Read the model definition and answer for the solid it produces. Units are mm, in the model's axes. Face numbers are marked on the shaded views. A direction names the side the tool comes from. Coordinates: 2 decimals unless noted, no trailing zeros. Loops run counter-clockwise (first coordinate to the right, second up) from the corner with the lowest first, then second, coordinate; pieces in that order, holes last. Notation, with made-up numbers: (-15.75, 6.5) - (41.25, 6.5) arc R8 cw to (41.25, 17.5) - close; hole circle Ø6 at (-11, 42). An arc over 180 degrees is marked (long way). Use one line per item in the form item = value. Start each with the question number.
1) A cutting plane is placed at A-A (z = 0). Give the vertices of the cut face in (x, y), and give its area (3 significant figures).
2) A cutting plane is placed at C-C (z = -12). Give the vertices of the cut face in (x, y).
3) Consider line 1 (X direction, y = -5.5, z = -16.5); line 2 (Z direction, x = 0, y = 1.4); line 3 (Y direction, x = 13, z = -13). Determine where each line is inside the solid, lowest interval first.
4) A cutting plane is placed at D-D (x = -5). Give the vertices of the cut face in (y, z), and give its area (3 significant figures).
5) A cutting plane is placed at B-B (y = -2). Give the vertices of the cut face in (x, z).
6) The mould has two halves that part along X. Classify the marked faces 1, 2, 3 and 4: released by +X, released by -X, zero draft, split by the parting line, or undercut.
7) Which of the six approach directions +Z, -Z, +X, -X, +Y, -Y give full straight-line access (tool end or side, diameter ignored) to the marked faces 5 and 6?
8) Each of these flat-tipped pins is pushed along its axis until it touches: P1, Ø2.5, axis at x = 14, z = -13, coming from the -Y side; P2, Ø4.5, axis at x = -13, y = -5.5, coming from the -Z side. Where does it stop, or does it pass through?
from build123d import *

# Parameters (mm, degrees)
F0_W     = 36
F0_H     = 37
F0_R     = 15
F1_DEPTH = 14
F0_R_2   = 12.5
F2_DEPTH = 3
F3_R     = 1.65
F4_DEPTH = 5
F5_R     = 2.5
F6_DEPTH = 8


with BuildPart() as f1:
    # F0 (on Front) → F1 (new body)
    with BuildSketch(Plane.XZ):
        with Locations((0, -0.5)):
            Rectangle(F0_W, F0_H)
        Circle(F0_R, mode=Mode.SUBTRACT)
    extrude(amount=F1_DEPTH)

    # F0 (on Front) → F2 (join)
    with BuildSketch(Plane.XZ):
        with Locations((0, -0.5)):
            Rectangle(F0_W, F0_H)
        Circle(F0_R, mode=Mode.SUBTRACT)
        Circle(F0_R)
        Circle(F0_R_2, mode=Mode.SUBTRACT)
    extrude(amount=-F2_DEPTH)

    # F3 (on face) → F4 (cut)
    with BuildSketch(Plane.XZ.offset(14)):
        with Locations((-14, 13)):
            Circle(F3_R)
        with Locations((-14, -13)):
            Circle(F3_R)
        with Locations((14, -13)):
            Circle(F3_R)
        with Locations((14, 13)):
            Circle(F3_R)
    extrude(amount=-F4_DEPTH, mode=Mode.SUBTRACT)

    # F5 (on face) → F6 (cut)
    with BuildSketch(Plane(origin=(0, 0, -19), x_dir=(1, 0, 0), z_dir=(0, 0, -1))):
        with Locations((-13, 5.5)):
            Circle(F5_R)
        with Locations((13, 5.5)):
            Circle(F5_R)
    extrude(amount=-F6_DEPTH, mode=Mode.SUBTRACT)


solid = f1.part
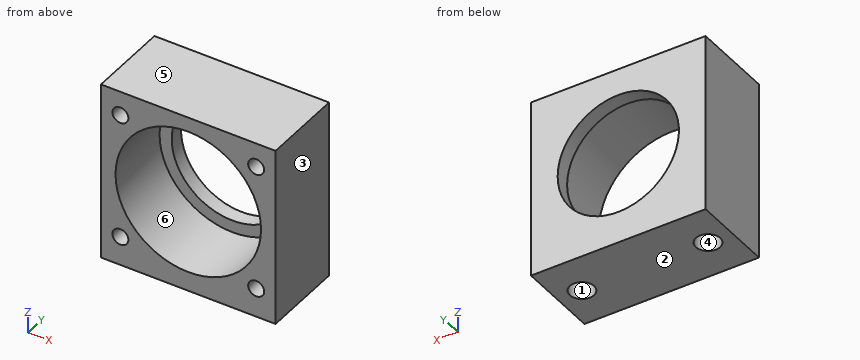
Found:
q1.outline = (-18, -14) - (-15, -14) - (-15, 0) - (-12.5, 0) - (-12.5, 3) - (-18, 3) - close; (12.5, 0) - (15, 0) - (15, -14) - (18, -14) - (18, 3) - (12.5, 3) - close
q1.area = 117 mm^2
q2.outline = (-18, -14) - (-15.31, -14) - (-15.31, -9) - (-12.69, -9) - (-12.69, -14) - (-9, -14) - (-9, 0) - (-3.5, 0) - (-3.5, 3) - (-18, 3) - close; (3.5, 0) - (9, 0) - (9, -14) - (12.69, -14) - (12.69, -9) - (15.31, -9) - (15.31, -14) - (18, -14) - (18, 3) - (3.5, 3) - close; hole circle Ø5 at (-13, -5.5); hole circle Ø5 at (13, -5.5)
q3.line_1 = -18 to -15.5, -10.5 to 10.5, 15.5 to 18
q3.line_2 = -19 to -12.5, 12.5 to 18
q3.line_3 = -9 to -8, -3 to 3
q4.outline = (-14, -19) - (3, -19) - (3, -11.46) - (0, -11.46) - (0, -14.14) - (-14, -14.14) - close; (-14, 14.14) - (0, 14.14) - (0, 11.46) - (3, 11.46) - (3, 18) - (-14, 18) - close
q4.area = 164 mm^2
q5.outline = (-18, -19) - (18, -19) - (18, 18) - (-18, 18) - close; hole circle Ø30 at (0, 0)
q6.face_1 = undercut
q6.face_2 = zero draft
q6.face_3 = released by +X
q6.face_4 = undercut
q7.face_5 = +Z, +X, -X, +Y, -Y
q7.face_6 = -Y
q8.P1 = -9
q8.P2 = -11
